Could you check a few things on this model? Use its own coordinates, in mm. A direction names the side the tool comes from. Round coordinates to 2 decimals unless told otherwise and drop trailing zeros. Write each loop counter-clockwise with the first axis right and the second up, starting at its lowest first coordinate (ties: lowest second). Pieces come first, ordered by that corner, then holes. Notation, with made-up numbers: (31, 85) -> (64, 85) arc R23 ccw to (64, 102) -> close; hole circle Ø5 at (73, 32). An arc over 180 degrees is marked (long way). Return JSON: item names as keys, results as strings.
from build123d import *

# Parameters (mm, degrees)
SKETCH1_W           = 28.5
SKETCH1_H           = 28.5
BOSS_EXTRUDE1_DEPTH = 7
FILLET1_R           = 2
SKETCH2_R           = 11
BOSS_EXTRUDE2_DEPTH = 1.6
SKETCH3_R           = 4
CUT_EXTRUDE1_DEPTH  = 1.6
SKETCH6_W           = 28.2
SKETCH6_H           = 28.2
BOSS_EXTRUDE4_DEPTH = 14
FILLET2_R           = 2
SKETCH7_W           = 28.5
SKETCH7_H           = 28.5
BOSS_EXTRUDE5_DEPTH = 7
FILLET3_R           = 2
SKETCH8_W           = 15
SKETCH8_H           = 5
BOSS_EXTRUDE6_DEPTH = 2.7
SKETCH9_R           = 1.4
CUT_EXTRUDE3_DEPTH  = 42.7
SKETCH10_R          = 3.5
CUT_EXTRUDE4_DEPTH  = 4
FILLET4_R           = 0.5
FILLET5_R           = 0.5
CUT_EXTRUDE5_START  = -0.1
SKETCH11_R          = 12
SKETCH11_R_2        = 11
CUT_EXTRUDE5_DEPTH  = 0.1
CUT_EXTRUDE6_START  = -2.5
SKETCH12_R          = 4
CUT_EXTRUDE6_DEPTH  = 2.5
SKETCH13_R          = 2.5
BOSS_EXTRUDE7_DEPTH = 0.5
FILLET6_R           = 0.2
SKETCH14_W          = 1
SKETCH14_H          = 1
CUT_EXTRUDE7_DEPTH  = 5
SKETCH_1_R          = 3
SHAFT_DEPTH         = 98


with BuildPart() as part:
    # Sketch1 → Boss-Extrude1 (new body)
    with BuildSketch(Plane.XY):
        Rectangle(SKETCH1_W, SKETCH1_H)
    extrude(amount=BOSS_EXTRUDE1_DEPTH)

    # Fillet1
    fillet1_edges = [part.edges().sort_by_distance(p)[0] for p in [
        (14.25, -14.25, 3.5),
        (-14.25, -14.25, 3.5),
        (-14.25, 14.25, 3.5),
        (14.25, 14.25, 3.5),
    ]]
    fillet(fillet1_edges, radius=FILLET1_R)

    # Sketch2 → Boss-Extrude2 (add)
    with BuildSketch(Plane.XY.offset(7)):
        Circle(SKETCH2_R)
    extrude(amount=BOSS_EXTRUDE2_DEPTH)

    # Sketch3 → Cut-Extrude1 (cut)
    with BuildSketch(Plane.XY.offset(8.6)):
        Circle(SKETCH3_R)
    extrude(amount=-CUT_EXTRUDE1_DEPTH, mode=Mode.SUBTRACT)

    # Sketch6 → Boss-Extrude4 (add)
    with BuildSketch(Plane(origin=(0, 0, 0), x_dir=(-1, 0, 0), z_dir=(0, 0, -1))):
        Rectangle(SKETCH6_W, SKETCH6_H)
    extrude(amount=BOSS_EXTRUDE4_DEPTH)

    # Fillet2
    # the kernel refuses this fillet: 2 mm, written as the material it takes off along each edge
    with BuildSketch(Plane(origin=(-14.1, -14.1, 0), x_dir=(0, 1, 0), z_dir=(0, 0, -1)), Plane(origin=(-14.1, 14.1, 0), x_dir=(1, 0, 0), z_dir=(0, 0, -1))) as fillet2_piece_1:
        with BuildLine():
            CenterArc((FILLET2_R, FILLET2_R), FILLET2_R, 180, 90)
            Line((0, FILLET2_R), (0, 0))
            Line((0, 0), (FILLET2_R, 0))
        make_face()
    extrude(amount=19, mode=Mode.SUBTRACT)
    with BuildSketch(Plane(origin=(14.1, 14.1, 0), x_dir=(-1, 0, 0), z_dir=(0, 0, -1)), Plane(origin=(14.1, -14.1, 0), x_dir=(0, 1, 0), z_dir=(0, 0, -1))) as fillet2_piece_2:
        with BuildLine():
            CenterArc((FILLET2_R, -FILLET2_R), FILLET2_R, 90, 90)
            Line((0, -FILLET2_R), (0, 0))
            Line((0, 0), (FILLET2_R, 0))
        make_face()
    extrude(amount=19, mode=Mode.SUBTRACT)

    # Sketch7 → Boss-Extrude5 (add)
    with BuildSketch(Plane(origin=(0, 0, -14), x_dir=(-1, 0, 0), z_dir=(0, 0, -1))):
        Rectangle(SKETCH7_W, SKETCH7_H)
    extrude(amount=BOSS_EXTRUDE5_DEPTH)

    # Fillet3
    fillet3_edges = [part.edges().sort_by_distance(p)[0] for p in [
        (-14.25, -14.25, -17.5),
        (-14.25, 14.25, -17.5),
        (14.25, 14.25, -17.5),
        (14.25, -14.25, -17.5),
    ]]
    fillet(fillet3_edges, radius=FILLET3_R)

    # Sketch8 → Boss-Extrude6 (add)
    with BuildSketch(Plane(origin=(0, 14.25, 0), x_dir=(1, 0, 0), z_dir=(0, 1, 0))):
        with Locations((0, 17)):
            Rectangle(SKETCH8_W, SKETCH8_H)
    extrude(amount=BOSS_EXTRUDE6_DEPTH)

    # Sketch9 → Cut-Extrude3 (cut)
    with BuildSketch(Plane.XY.offset(7)):
        with Locations((-11.5, 11.5)):
            Circle(SKETCH9_R)
        with Locations((11.5, 11.5)):
            Circle(SKETCH9_R)
        with Locations((11.5, -11.5)):
            Circle(SKETCH9_R)
        with Locations((-11.5, -11.5)):
            Circle(SKETCH9_R)
    extrude(amount=-CUT_EXTRUDE3_DEPTH, mode=Mode.SUBTRACT)

    # Sketch10 → Cut-Extrude4 (cut)
    with BuildSketch(Plane(origin=(0, 0, -21), x_dir=(-1, 0, 0), z_dir=(0, 0, -1))):
        with Locations((-11.5, 11.5)):
            Circle(SKETCH10_R)
        with Locations((11.5, 11.5)):
            Circle(SKETCH10_R)
        with Locations((11.5, -11.5)):
            Circle(SKETCH10_R)
        with Locations((-11.5, -11.5)):
            Circle(SKETCH10_R)
    extrude(amount=-CUT_EXTRUDE4_DEPTH, mode=Mode.SUBTRACT)

    # Fillet4
    fillet4_edges = [part.edges().sort_by_distance(p)[0] for p in [
        (14.25, -9.334936491, -19),
        (9.334936491, -14.25, -19),
        (-14.25, -9.334936491, -19),
        (-9.334936491, -14.25, -19),
        (-9.334936491, 14.25, -19),
        (-14.25, 9.334936491, -19),
        (9.334936491, 14.25, -19),
        (14.25, 9.334936491, -19),
    ]]
    fillet(fillet4_edges, radius=FILLET4_R)

    # Fillet5
    fillet5_edges = [part.edges().sort_by_distance(p)[0] for p in [
        (-14.25, 0, -21),
        (9.025126266, -9.025126266, -21),
        (0, -14.25, -21),
        (-9.025126266, -9.025126266, -21),
        (-9.025126266, 9.025126266, -21),
        (0, 14.25, -21),
        (9.025126266, 9.025126266, -21),
        (14.25, 0, -21),
        (13.983853587, 8.634752599, -21),
        (8.634752599, 13.983853587, -21),
        (13.983853587, -8.634752599, -21),
        (8.634752599, -13.983853587, -21),
        (-8.634752599, -13.983853587, -21),
        (-13.983853587, -8.634752599, -21),
        (-8.634752599, 13.983853587, -21),
        (-13.983853587, 8.634752599, -21),
    ]]
    fillet(fillet5_edges, radius=FILLET5_R)

    # Sketch11 → Cut-Extrude5 (cut)
    with BuildSketch(Plane.XY.offset(7).offset(CUT_EXTRUDE5_START)):
        Circle(SKETCH11_R)
        Circle(SKETCH11_R_2, mode=Mode.SUBTRACT)
    extrude(amount=CUT_EXTRUDE5_DEPTH, mode=Mode.SUBTRACT)

    # Sketch12 → Cut-Extrude6 (cut)
    with BuildSketch(Plane(origin=(0, 0, -21), x_dir=(-1, 0, 0), z_dir=(0, 0, -1)).offset(CUT_EXTRUDE6_START)):
        with Locations(Location((0, 0, 0), (0, 0, 180))):
            Circle(SKETCH12_R)
    extrude(amount=CUT_EXTRUDE6_DEPTH, mode=Mode.SUBTRACT)

    # Sketch13 → Boss-Extrude7 (add)
    with BuildSketch(Plane(origin=(0, 0, -18.5), x_dir=(-1, 0, 0), z_dir=(0, 0, -1))):
        Circle(SKETCH13_R)
    extrude(amount=BOSS_EXTRUDE7_DEPTH)

    # Fillet6
    fillet6_edges = [part.edges().sort_by_distance(p)[0] for p in [
        (2.5, 0, -19),
    ]]
    fillet(fillet6_edges, radius=FILLET6_R)

    # Sketch14 → Cut-Extrude7 (cut)
    with BuildSketch(Plane(origin=(0, 16.95, 0), x_dir=(1, 0, 0), z_dir=(0, 1, 0))):
        with Locations((-6.3, 17)):
            Rectangle(SKETCH14_W, SKETCH14_H)
        with Locations((-3.76, 17)):
            Rectangle(SKETCH14_W, SKETCH14_H)
        with Locations((-1.22, 17)):
            Rectangle(SKETCH14_W, SKETCH14_H)
        with Locations((1.32, 17)):
            Rectangle(SKETCH14_W, SKETCH14_H)
        with Locations((3.86, 17)):
            Rectangle(SKETCH14_W, SKETCH14_H)
        with Locations((6.4, 17)):
            Rectangle(SKETCH14_W, SKETCH14_H)
    extrude(amount=-CUT_EXTRUDE7_DEPTH, mode=Mode.SUBTRACT)

    # Эскиз1 → Shaft (add)
    with BuildSketch(Plane.XY.offset(7)):
        Circle(SKETCH_1_R)
    extrude(amount=SHAFT_DEPTH)


solid = part.part
1) I want a section at B-B, the plane z = 85. Please give me the cut outline in (x, y), and give its area (3 significant figures).
Return value:
{"outline": "circle Ø6 at (0, 0)", "area": "28.3 mm²"}
2) I want a section at A-A, the plane y = -6. Please give me the cut outline in (x, z), and give its area (3 significant figures).
Return value:
{"outline": "(-14.25, -20.5) arc R0.5 ccw to (-13.75, -21) -> (13.75, -21) arc R0.5 ccw to (14.25, -20.5) -> (14.25, -14) -> (14.1, -14) -> (14.1, 0) -> (14.25, 0) -> (14.25, 7) -> (10.39, 7) -> (10.39, 6.9) -> (9.22, 6.9) -> (9.22, 8.6) -> (-9.22, 8.6) -> (-9.22, 6.9) -> (-10.39, 6.9) -> (-10.39, 7) -> (-14.25, 7) -> (-14.25, 0) -> (-14.1, 0) -> (-14.1, -14) -> (-14.25, -14) -> close", "area": "823 mm²"}
3) Will these pins go through, and if not, where does the flat tip stop? pin 1 Ø1 at (x, y) = (9.5, 10.5) entering from +Z; pin 2 Ø6 at (x, y) = (-6, 3) entering from +Z; pin 3 Ø2 at (x, z) = (-4, -5) entering from -Y.
Return value:
{"pin 1": "z = 7", "pin 2": "z = 8.6", "pin 3": "y = -14.1"}
4) If I drill on probe 1 along Y at (x, z) = (11.5, -10.5); probe 2 along Y at (x, z) = (0, 7.45); probe 3 along Z at (x, y) = (-5, 15), over which ranges is the centre line in solid material (lowest first)? Write a range as [from, to].
Return value:
{"probe 1": "[-14.1, -12.9], [-10.1, 10.1], [12.9, 14.1]", "probe 2": "[-11, -4], [-3, 3], [4, 11]", "probe 3": "[-19.5, -14.5]"}
5) Thinking about a two-plate mould opening in Z: for faces 5 (the face through (0, -14.1, -7)), 6 (the face through (-14.25, 0, 3)), 7 (the face through (-10, 10, -17)), which applies, pulls with the +Z half, pulls with the -Z half, needs draft (parallel to the pull), parting line crosses it, or undercut?
Return value:
{"face 5": "undercut", "face 6": "needs draft", "face 7": "pulls with the -Z half"}
6) For faces 1 (the face through (-14.1, 0, -7)), 2 (the face through (-9.07, -8.98, -18.77)), 3 (the face through (13.53, -13.5, -6.9)), 4 (the face through (5, -10, 6.9)), which set-ups out of +Z, -Z, +X, -X, +Y, -Y let a thin tool reach every point of the face, with its end or its side?
Return value:
{"face 1": "-X, +Y, -Y", "face 2": "-Z", "face 3": "+X, -Y", "face 4": "+Z"}
